Check sheet for the modelled part. Datum: model origin and axes. Units: mm. Face numbers are marked on the shaded views. A direction names the side the tool comes from. Coordinates: 2 decimals unless noted, no trailing zeros. Order: outer loops, then holes, each group sorted by start corner. A loop starts at its lowest first (then second) coordinate and runs counter-clockwise, first axis right, second up.
1. Thickness scan on line 1 (X direction, y = 11.75, z = 0.5); line 2 (X direction, y = 2, z = 2.7); line 3 (Y direction, x = -2, z = 1.7). Record the ranges inside material, lowest first.
2. Cross-section at C-C (y = 7). Enter the section's corners in (x, z), then the cut area to 3 significant figures.
3. Cross-section at A-A (y = 4.25). Enter the section's corners in (x, z).
4. Cross-section at D-D (z = 0.5). Enter the section's corners in (x, y), then the cut area to 3 significant figures.
5. Draft check along X on the marked faces 1, 2, 3 and 4. Enter one of: released by +X, released by -X, zero draft, split by the parting line, or undercut.
6. Set-up check for the marked faces 5 and 6: record each of +Z, -Z, +X, -X, +Y, -Y from which the full face is reachable in a straight line by a thin tool's end or side.
7. Gauge pin test, flat ends, axial feed: pin 1 Ø1 at (x, z) = (1, 0.5) entering from +Y; pin 2 Ø8 at (x, y) = (-4.5, 6.5) entering from -Z; pin 3 Ø0.9 at (y, z) = (5, 1.5) entering from -X; pin 4 Ø1.5 at (y, z) = (6.5, 1) entering from +X. Record the tip position at first contact, or that the pin passes through.
```python
from build123d import *

# Parameters (mm, degrees)
F1_DEPTH    = 3
F3_DEPTH    = 2
F4_R        = 1.49999
F5_T1_DEPTH = 3
F6_T1_DEPTH = 30.4128784748


# Not quite as in the source:
# - a fillet or chamfer that OpenCascade refuses, or shapes differently, is made with other operations: its cross-section is extruded or revolved along the edge and cut away or added
# - a fillet or chamfer is up to 0.001 mm smaller than in the source, because OpenCascade refuses the exact size
# - a feature names something its author has since deleted; it is built from what else it names


with BuildPart() as f1:
    # F0 (on Top) → F1 (new body)
    with BuildSketch(Plane.XY):
        Polygon((-7.5, 12.5), (-7.5, -12.5), (0, -12.5), (0, 12.5), (-3.5, 12.5), (-3.5, 2.5), (-5.5, 2.5), (-5.5, 12.5), align=None)
    extrude(amount=F1_DEPTH)

    # F2 (on face) → F3 (join)
    with BuildSketch(Plane(origin=(-7.5, 0, 0), x_dir=(0, -1, 0), z_dir=(-1, 0, 0))):
        with BuildLine():
            ThreePointArc((-10.4999999883, 3), (-11.2071067853, 1.2928932229), (-9.5, 2))
            ThreePointArc((-9.5, 2), (-9.7928932147, 2.7071067771), (-10.4999999883, 3))
        make_face()
    extrude(amount=F3_DEPTH)

    # F4 (radius 1.5 in the source; OpenCascade refuses exactly that, so slightly less here)
    f4_edges = [f1.edges().sort_by_distance(p)[0] for p in [
        (-6.5, 12.5, 0),
        (-6.5, 12.5, 3),
        (-1.75, 12.5, 0),
        (-1.75, 12.5, 3),
    ]]
    fillet(f4_edges, radius=F4_R)

    # F5: fillet of radius 4 on 1 edges, made by hand

    # F5_s2 → F5_t1 (join)
    with BuildSketch(Plane.XY):
        with BuildLine():
            ThreePointArc((-5.5, 5.9641016151), (-4.9641016151, 3.9641016151), (-3.5, 2.5))
            Line((-3.5, 2.5), (-5.5, 2.5))
            Line((-5.5, 2.5), (-5.5, 5.9641016151))
        make_face()
    extrude(amount=F5_T1_DEPTH)

    # F6: fillet of radius 5 on 1 edges, made by hand

    # F6_s2 → F6_t1 (cut)
    with BuildSketch(Plane.YZ.offset(-18.9564392374)):
        with BuildLine():
            ThreePointArc((-7.917424305, 0), (-10.6560370926, 0.8166998673), (-12.5, 3))
            Line((-12.5, 3), (-12.5, 0))
            Line((-12.5, 0), (-7.917424305, 0))
        make_face()
    extrude(amount=F6_T1_DEPTH, mode=Mode.SUBTRACT)

    # F7: F1 across face


with BuildPart() as f1_1:
    add(f1.part)
    add(f1.part.mirror(Plane(origin=(0, 0.4580070694, 1.5370600849), x_dir=(0, 1, 0), z_dir=(1, 0, 0))))


solid = f1_1.part
```
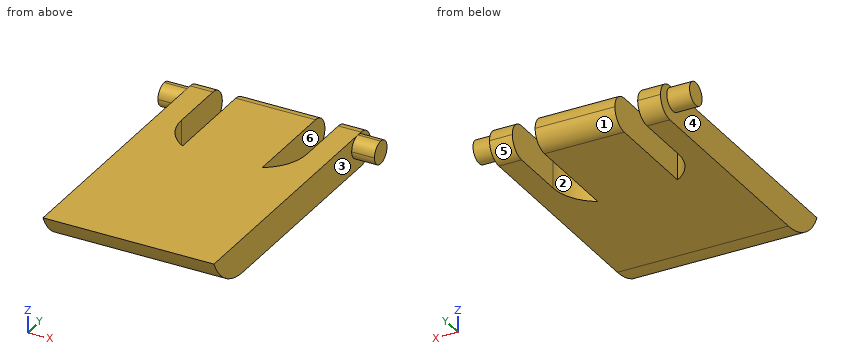
Data:
1. line 1: x = -7.5 to -5.5, -3.5 to 3.5, 5.5 to 7.5
1. line 2: x = -7.5 to 7.5
1. line 3: y = -11.67 to 12.49
2. outline: (-7.5, 0) - (-5.5, 0) - (-5.5, 3) - (-7.5, 3) - close; (-3.5, 0) - (3.5, 0) - (3.5, 3) - (-3.5, 3) - close; (5.5, 0) - (7.5, 0) - (7.5, 3) - (5.5, 3) - close
2. area: 33.0 mm2
3. outline: (-7.5, 0) - (-5.11, 0) - (-5.11, 3) - (-7.5, 3) - close; (-3.5, 0) - (3.5, 0) - (3.5, 3) - (-3.5, 3) - close; (5.11, 0) - (7.5, 0) - (7.5, 3) - (5.11, 3) - close
4. outline: (-7.5, -10.1) - (7.5, -10.1) - (7.5, 12.12) - (5.5, 12.12) - (5.5, 5.96) arc R4 cw to (3.5, 2.5) - (3.5, 12.12) - (-3.5, 12.12) - (-3.5, 2.5) arc R4 cw to (-5.5, 5.96) - (-5.5, 12.12) - (-7.5, 12.12) - close
4. area: 299 mm2
5. face 1: zero draft
5. face 2: undercut
5. face 3: released by +X
5. face 4: released by -X
6. face 5: -Z, +X, -X, +Y
6. face 6: +Z, -Z, +Y
7. pin 1: stops at y = 12.41
7. pin 2: stops at z = 0
7. pin 3: stops at x = -7.5
7. pin 4: stops at x = 7.5
